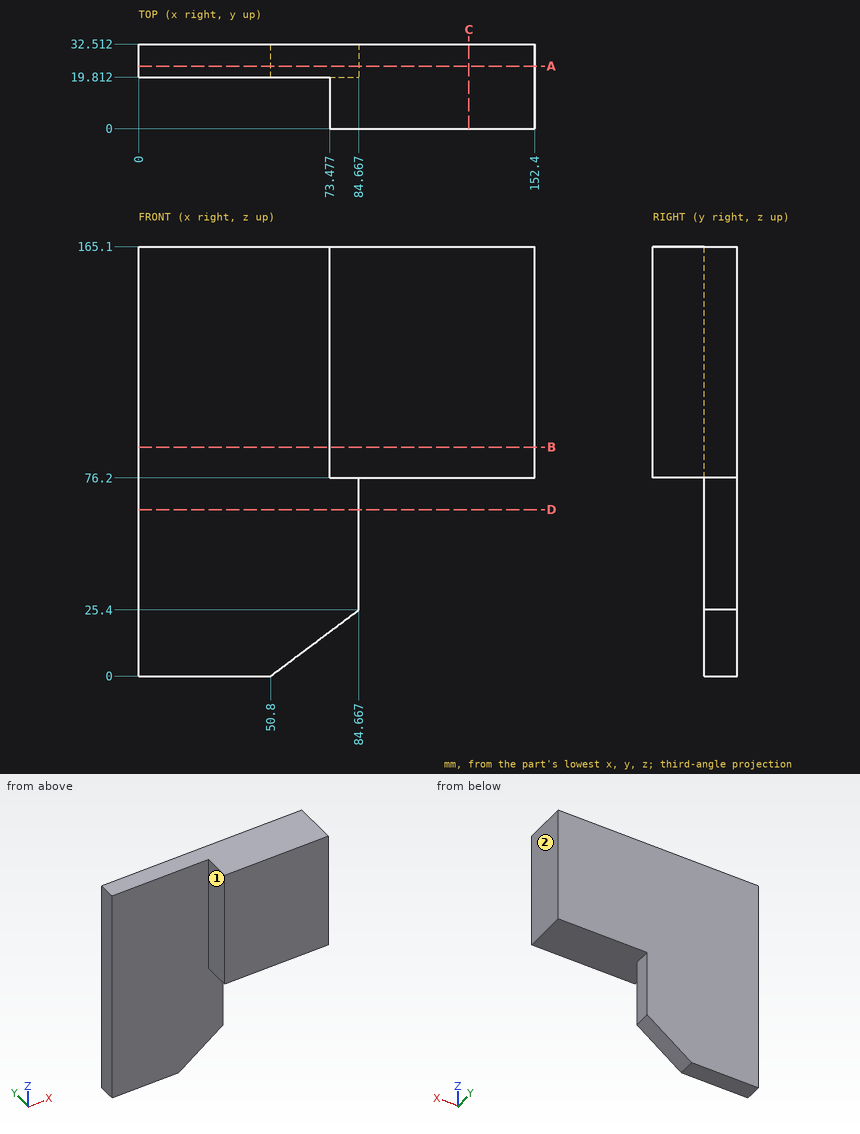
Source: three-view drawing plus pictorial views. Frame: mm from the lowest corner of the part. A direction names the side the tool comes from. Round coordinates to 2 decimals unless told otherwise and drop trailing zeros. Order: outer loops, then holes, each group sorted by start corner. A loop starts at its lowest first (then second) coordinate and runs counter-clockwise, first axis right, second up. Notation, with made-up numbers: (-18, 26.25) - (18, 26.25) arc R15 cw to (18, 40.25) - close; hole circle Ø11 at (-23.5, 28). An arc over 180 degrees is marked (long way). Answer in a Markdown table with one row per item.
Item 1: Section query B-B (z = 88). Return the cut outline in (x, y).
Model answer:
| item | result |
|---|---|
| outline | (0, 19.81) - (73.48, 19.81) - (73.48, 0) - (152.4, 0) - (152.4, 32.51) - (0, 32.51) - close |
Item 2: Pin query (flat end, axial travel): pin 1 (12 mm diameter, centred on y = 12.5, z = 89.5, fed in from -X); pin 2 (6.5 mm diameter, centred on y = 24.5, z = 38, fed in from +X); pin 3 (16.5 mm diameter, centred on x = 116, y = 9.5, fed in from -Z). Return the tip coordinate at first contact, or that it passes through.
Model answer:
| item | result |
|---|---|
| pin 1 | stops at x = 73.48 |
| pin 2 | stops at x = 84.67 |
| pin 3 | stops at z = 76.2 |
Item 3: Line query: line 1 (Y direction, x = 45, z = 83.5); line 2 (X direction, y = 12, z = 95); line 3 (Z direction, x = 135, y = 6.5). Output: solid intervals per line, ascending.
Model answer:
| item | result |
|---|---|
| line 1 | y = 19.81 to 32.51 |
| line 2 | x = 73.48 to 152.4 |
| line 3 | z = 76.2 to 165.1 |
Item 4: Section query D-D (z = 64). Return the cut outline in (x, y), then the cut area to 3 significant figures.
Model answer:
| item | result |
|---|---|
| outline | (0, 19.81) - (84.67, 19.81) - (84.67, 32.51) - (0, 32.51) - close |
| area | 1,080 mm² |
Item 5: Section query A-A (y = 24). Return the cut outline in (x, z), then the cut area to 3 significant figures.
Model answer:
| item | result |
|---|---|
| outline | (0, 0) - (50.8, 0) - (84.67, 25.4) - (84.67, 76.2) - (152.4, 76.2) - (152.4, 165.1) - (0, 165.1) - close |
| area | 19,600 mm² |
Item 6: Section query C-C (x = 127). Return the cut outline in (y, z).
Model answer:
| item | result |
|---|---|
| outline | (0, 76.2) - (32.51, 76.2) - (32.51, 165.1) - (0, 165.1) - close |
Item 7: Reachability of the marked faces 1 and 2 from +Z, -Z, +X, -X, +Y, -Y: full face, straight path, thin tool, end or side. Return the list, or none.
Model answer:
| item | result |
|---|---|
| face 1 | +Z, -Z, -X, -Y |
| face 2 | +Z, -Z, +X, +Y, -Y |
